from build123d import *

# Parameters (mm, degrees)
SKETCH1_W           = 130
SKETCH1_H           = 120
BOSS_EXTRUDE1_DEPTH = 4
SKETCH2_R           = 12.7
SKETCH2_R_2         = 5.08
CUT_EXTRUDE1_DEPTH  = 89.549421229
BOSS_EXTRUDE2_START = -4
SKETCH3_W           = 130
SKETCH3_H           = 4
BOSS_EXTRUDE2_DEPTH = 50
SKETCH5_R           = 5
CUT_EXTRUDE2_DEPTH  = 143.059846544


with BuildPart() as part:
    # Sketch1 → Boss-Extrude1 (new body)
    with BuildSketch(Plane.XY):
        Rectangle(SKETCH1_W, SKETCH1_H)
    extrude(amount=BOSS_EXTRUDE1_DEPTH)

    # Sketch2 → Cut-Extrude1 (cut, through all)
    with BuildSketch(Plane.XY.offset(4)):
        with Locations((-40, 15)):
            Circle(SKETCH2_R)
        with Locations((-40, 43.575)):
            Circle(SKETCH2_R_2)
        with Locations(Location((-40, -13.575, 0), (0, 0, 180))):
            Circle(SKETCH2_R_2)
        with Locations((40, -13.575)):
            Circle(SKETCH2_R_2)
        with Locations(Location((40, 15, 0), (0, 0, 180))):
            Circle(SKETCH2_R)
        with Locations(Location((40, 43.575, 0), (0, 0, 180))):
            Circle(SKETCH2_R_2)
    extrude(amount=-CUT_EXTRUDE1_DEPTH, mode=Mode.SUBTRACT)

    # Sketch3 → Boss-Extrude2 (add)
    with BuildSketch(Plane.XY.offset(4).offset(BOSS_EXTRUDE2_START)):
        with Locations((0, -58)):
            Rectangle(SKETCH3_W, SKETCH3_H)
    extrude(amount=BOSS_EXTRUDE2_DEPTH)

    # Sketch5 → Cut-Extrude2 (cut, through all)
    with BuildSketch(Plane(origin=(0, -56, 0), x_dir=(1, 0, 0), z_dir=(0, 1, 0))):
        with Locations(Location((-55, -14, 0), (0, 0, 270))):
            Circle(SKETCH5_R)
        with Locations(Location((-55, -40, 0), (0, 0, 270))):
            Circle(SKETCH5_R)
    cut_extrude2 = extrude(amount=-CUT_EXTRUDE2_DEPTH, mode=Mode.SUBTRACT)

    # Mirror1: Cut-Extrude2 across plane
    add(cut_extrude2.mirror(Plane(origin=(0, 0, 0), x_dir=(0, 0, 1), z_dir=(1, 0, 0))), mode=Mode.SUBTRACT)


solid = part.part
Design review of the part built by this model. Coordinates are the model's own, in mm. A direction names the side the tool comes from. Round coordinates to 2 decimals unless told otherwise and drop trailing zeros. Write each loop counter-clockwise with the first axis right and the second up, starting at its lowest first coordinate (ties: lowest second). Pieces come first, ordered by that corner, then holes.
Item 1: Consider section D-D on x = -14. Give the boundary of the cut face in (y, z).
Item 2: Consider section C-C on y = 16.5. Give the boundary of the cut face in (x, z).
Item 3: Consider section B-B on x = 40. Give the boundary of the cut face in (y, z) (3 decimals), and give its area (3 significant figures).
Item 4: For pin 1 Ø10 at (x, y) = (-24.5, -20) entering from +Z; pin 2 Ø23 at (x, z) = (-31.5, 36) entering from +Y, all flat-tipped, find the tip position at first contact; note any pin that passes through.
Item 5: Draft analysis for pull direction X (two halves, no side actions). For faces 1 (the flat face through (65, -18, 3)), 2 (the cylindrical face through (-44.693, -11.629, 2.028)), 3 (the flat face through (-1, -60, 25)), 4 (the flat face through (-65, -18, 3)), state which applies: released by +X, released by -X, zero draft, split by the parting line, or undercut.
Item 6: Wall thickness on L1, parallel to Y at x = -40, z = 2.1 (3 decimals); L2, parallel to X at y = -57.2, z = 14; L3, parallel to Y at x = -20.5, z = 6: over which ranges is each line inside the solid? List them lowest first.
Item 7: For faces 5 (the cylindrical face through (44.7, -15.5, 2)), 6 (the flat face through (-1, -56, 27)), list the 3-axis set-ups (+Z, -Z, +X, -X, +Y, -Y) from which the entire face can be reached by the end or side of a thin tool; tool diameter is ignored.
Item 8: Consider section A-A on z = 43. Give the boundary of the cut face in (x, y), and give its area (3 significant figures).
Check values:
1. outline: (-60, 0) - (60, 0) - (60, 4) - (-56, 4) - (-56, 50) - (-60, 50) - close
2. outline: (-65, 0) - (-52.61, 0) - (-52.61, 4) - (-65, 4) - close; (-27.39, 0) - (27.39, 0) - (27.39, 4) - (-27.39, 4) - close; (52.61, 0) - (65, 0) - (65, 4) - (52.61, 4) - close
3. outline: (-60, 0) - (-18.655, 0) - (-18.655, 4) - (-56, 4) - (-56, 50) - (-60, 50) - close; (-8.495, 0) - (2.3, 0) - (2.3, 4) - (-8.495, 4) - close; (27.7, 0) - (38.495, 0) - (38.495, 4) - (27.7, 4) - close; (48.655, 0) - (60, 0) - (60, 4) - (48.655, 4) - close
3. area: 481 mm2
4. pin 1: stops at z = 4
4. pin 2: stops at y = -56
5. face 1: released by +X
5. face 2: undercut
5. face 3: zero draft
5. face 4: released by -X
6. L1: y = -60 to -18.655, -8.495 to 2.3, 27.7 to 38.495, 48.655 to 60
6. L2: x = -65 to -60, -50 to 50, 60 to 65
6. L3: y = -60 to -56
7. face 5: +Z, -Z
7. face 6: +Z, +X, -X, +Y
8. outline: (-65, -60) - (-59, -60) - (-59, -56) - (-65, -56) - close; (-51, -60) - (51, -60) - (51, -56) - (-51, -56) - close; (59, -60) - (65, -60) - (65, -56) - (59, -56) - close
8. area: 456 mm2
